from build123d import *

# Parameters (mm, degrees)
SKETCH1_R           = 5.25
BOSS_EXTRUDE1_DEPTH = 5.5
SKETCH2_R           = 4
BOSS_EXTRUDE2_DEPTH = 1.7
FILLET1_R           = 0.15
SKETCH3_R           = 7.5
BOSS_EXTRUDE3_DEPTH = 5
SKETCH4_R           = 2.55
CUT_EXTRUDE1_DEPTH  = 3
CUT_EXTRUDE2_DEPTH  = 4.7
FILLET2_R           = 2
FILLET3_R           = 1
FILLET4_R           = 1


with BuildPart() as part:
    # Sketch1 → Boss-Extrude1 (new body)
    with BuildSketch(Plane(origin=(0, 0, 0), x_dir=(1, 0, 0), z_dir=(0, 1, 0))):
        with Locations(Location((0, 0, 0), (0, 0, 270))):
            Circle(SKETCH1_R)
    extrude(amount=BOSS_EXTRUDE1_DEPTH)

    # Sketch2 → Boss-Extrude2 (add)
    with BuildSketch(Plane.XZ):
        with Locations(Location((0, 0, 0), (0, 0, 270))):
            Circle(SKETCH2_R)
    extrude(amount=BOSS_EXTRUDE2_DEPTH)

    # Fillet1
    fillet1_edges = [part.edges().sort_by_distance(p)[0] for p in [
        (0, 0, 4),
    ]]
    fillet(fillet1_edges, radius=FILLET1_R)

    # Sketch3 → Boss-Extrude3 (add)
    with BuildSketch(Plane(origin=(0, 5.5, 0), x_dir=(1, 0, 0), z_dir=(0, 1, 0))):
        with Locations(Location((0, 0, 0), (0, 0, 270))):
            Circle(SKETCH3_R)
    extrude(amount=BOSS_EXTRUDE3_DEPTH)

    # Sketch4 → Cut-Extrude1 (cut)
    with BuildSketch(Plane(origin=(0, 10.5, 0), x_dir=(1, 0, 0), z_dir=(0, 1, 0))):
        with Locations(Location((0, 0, 0), (0, 0, 270))):
            Circle(SKETCH4_R)
    extrude(amount=-CUT_EXTRUDE1_DEPTH, mode=Mode.SUBTRACT)

    # Sketch5 → Cut-Extrude2 (cut)
    with BuildSketch(Plane.XZ.offset(1.7)):
        Polygon((2.713546265, 0), (1.356773133, 2.35), (-1.356773133, 2.35), (-2.713546265, 0), (-1.356773133, -2.35), (1.356773133, -2.35), align=None)
    extrude(amount=-CUT_EXTRUDE2_DEPTH, mode=Mode.SUBTRACT)

    # Fillet2
    fillet2_edges = [part.edges().sort_by_distance(p)[0] for p in [
        (0, 5.5, -5.25),
    ]]
    fillet(fillet2_edges, radius=FILLET2_R)

    # Fillet3
    fillet3_edges = [part.edges().sort_by_distance(p)[0] for p in [
        (0, 0, -5.25),
    ]]
    fillet(fillet3_edges, radius=FILLET3_R)

    # Fillet4
    fillet4_edges = [part.edges().sort_by_distance(p)[0] for p in [
        (0, 5.5, -7.5),
    ]]
    fillet(fillet4_edges, radius=FILLET4_R)


solid = part.part
Work out the finished part from the listing and answer in its coordinate system (mm). A direction names the side the tool comes from. Round coordinates to 2 decimals unless told otherwise and drop trailing zeros. Order: outer loops, then holes, each group sorted by start corner. A loop starts at its lowest first (then second) coordinate and runs counter-clockwise, first axis right, second up. Notation, with made-up numbers: M 37.25,46.25 L 41.25,46.25 A22 ccw 41.25,65.25 Z; hole C 69,-27.5 d10. An arc over 180 degrees is marked long. Put each result on its own line as item: value. Start each with the question number.
Q1. Section A-A, the plane y = -0.5 is taken. Write down the section's boundary in (x, z), and give its area (3 significant figures).
Q2. For a pull along X with two mould halves and no side action, classify faces 4 (the flat face through (0, 7.5, 0)), 5 (the flat face through (0, 10.5, 3)), 6 (the cylindrical face through (0.33, 8.424, -7.493)) as pulls with the +X half, pulls with the -X half, needs draft (parallel to the pull), parting line crosses it, or undercut.
Q3. Flat-ended cylindrical pins translate along their axes: pin 1 (3 mm diameter, centred on x = 0.5, y = -0.5, fed in from -Z); pin 2 (5 mm diameter, centred on y = 8.5, z = -4.5, fed in from -X); pin 3 (5 mm diameter, centred on y = 9, z = -4, fed in from +X). Find the tip coordinate at first contact, or state that the pin passes through.
Q4. Straight lines are drawn through the part: L1, parallel to X at y = 8.9, z = 0; L2, parallel to Y at x = -0.75, z = 2.25; L3, parallel to Z at x = -1.75, y = -0.5. For each, find the intervals that lie inside material, in ascending order. Write a range as [from, to].
Q5. A tool of negligible diameter and unlimited length cuts with its end or side. For faces 1 (the cylindrical face through (0.77, 9.02, 2.43)), 2 (the flat face through (-2.026, 0.617, 1.191)), 3 (the flat face through (-2, -1.7, -2)), from which of +Z, -Z, +X, -X, +Y, -Y can it reach the whole face along a straight path? Write none if from no direction.
Findings below:
1. outline: C 0,0 d8; hole M -2.71,0 L -1.36,-2.35 L 1.36,-2.35 L 2.71,0 L 1.36,2.35 L -1.36,2.35 Z
1. area: 31.1 mm^2
2. face 4: undercut
2. face 5: needs draft
2. face 6: parting line crosses it
3. pin 1: stops at z = -5.25
3. pin 2: stops at x = -7.23
3. pin 3: stops at x = 7.35
4. L1: x = [-7.5, -2.55], [2.55, 7.5]
4. L2: y = [3, 7.5]
4. L3: z = [-3.6, -1.67], [1.67, 3.6]
5. face 1: +Y
5. face 2: -Y
5. face 3: +Z, -Z, +X, -X, -Y
